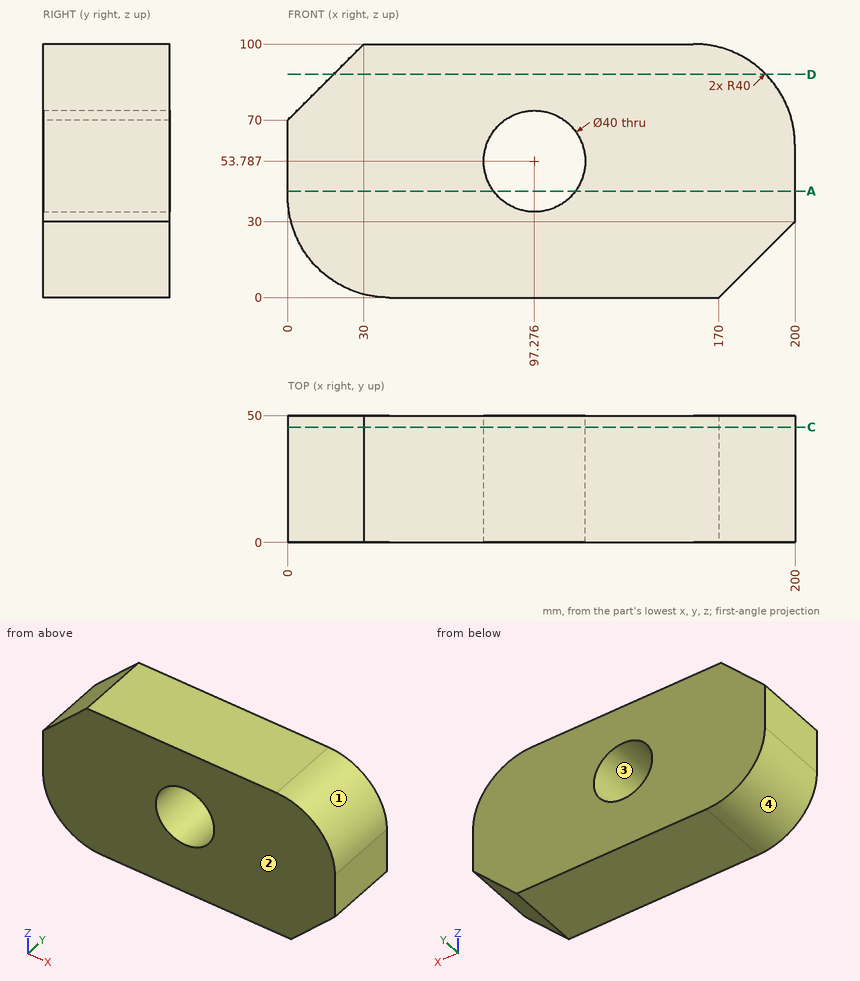
Could you check a few things on this drawing? It's one solid part, dimensions in mm from its lowest x, y, z. Round coordinates to 2 decimals unless told otherwise and drop trailing zeros. Loops run counter-clockwise (first coordinate to the right, second up) from the corner with the lowest first, then second, coordinate; pieces in that order, holes last. Notation, with made-up numbers: M -28,59 L -1,59 A19 ccw -1,76 Z; hole C 37,85.25 d2. An arc over 180 degrees is marked long. Write each question's results on one line, items separated by ' | '. Start each with the question number.
(1) I want a section at A-A (z = 42). Please give me the cut outline in (x, y), then the cut area to 3 significant figures.
(2) If I drill on probe 1 along X at (y, z) = (36, 52); probe 2 along Z at (x, y) = (82, 17) (1 decimal); probe 3 along Z at (x, y) = (101, 13.5), over which ranges is the centre line in solid material (lowest first)? Write a range as from..to.
(3) I want a section at C-C (y = 45.5). Please give me the cut outline in (x, z), then the cut area to 3 significant figures.
(4) Will these pins go through, and if not, where does the flat tip stop? P1, Ø12, axis at y = 24, z = 15.5, coming from the -X side (1 decimal); P2, Ø12, axis at x = 174, y = 19.5, coming from the +Z side.
(5) Thinking about a two-plate mould opening in Z: for the marked faces 1, 2, 3 and 4, which applies, pulls with the +Z half, pulls with the -Z half, needs draft (parallel to the pull), parting line crosses it, or undercut?
(6) I want a section at D-D (z = 88). Please give me the cut outline in (x, y), then the cut area to 3 significant figures.
Solved:
1) outline: M 0,0 L 81.12,0 L 81.12,50 L 0,50 Z; M 113.43,0 L 200,0 L 200,50 L 113.43,50 Z | area: 8,380 mm²
2) probe 1: x = 0..77.36, 117.2..200 | probe 2: z = 0..40.9, 66.7..100 | probe 3: z = 0..34.14, 73.44..100
3) outline: M 0,40 A40 ccw 40,0 L 170,0 L 200,30 L 200,60 A40 ccw 160,100 L 30,100 L 0,70 Z; hole C 97.28,53.79 d40 | area: 17,200 mm²
4) P1: stops at x = 4.5 | P2: stops at z = 99.19
5) face 1: pulls with the +Z half | face 2: needs draft | face 3: undercut | face 4: pulls with the -Z half
6) outline: M 18,0 L 188.57,0 L 188.57,50 L 18,50 Z | area: 8,530 mm²
